CAD build for the part. Positions are in the model's coordinates, mm. Coordinates: 2 decimals unless noted, no trailing zeros. Order: outer loops, then holes, each group sorted by start corner. A loop starts at its lowest first (then second) coordinate and runs counter-clockwise, first axis right, second up. Notation, with made-up numbers: M -21,89.25 L 19,89.25 A27 ccw 19,107.25 Z; hole C 2,-39 d11. An arc over 180 degrees is marked long. Write item = value, one per line.
from build123d import *

# Parameters (mm, degrees)
SKETCH1_R           = 1.55
BOSS_EXTRUDE1_DEPTH = 5
FILLET1_R           = 1
SKETCH2_R           = 2.9
CUT_EXTRUDE1_DEPTH  = 3


with BuildPart() as part:
    # Sketch1 → Boss-Extrude1 (new body)
    with BuildSketch(Plane(origin=(0, 0, 0), x_dir=(1, 0, 0), z_dir=(0, 1, 0))):
        with BuildLine():
            ThreePointArc((-29.5, 4), (-33.5, 0), (-29.5, -4))
            ThreePointArc((-29.5, -4), (-16.900654795, -5.373538993), (-4.893229568, -9.429626812))
            ThreePointArc((-4.893229568, -9.429626812), (14.756477238, -11.986867848), (32.328427125, -2.828427125))
            ThreePointArc((32.328427125, -2.828427125), (32.328427125, 2.828427125), (26.671572875, 2.828427125))
            ThreePointArc((26.671572875, 2.828427125), (13.359489628, -4.109785544), (-1.526651892, -2.172481729))
            ThreePointArc((-1.526651892, -2.172481729), (-15.176874162, 2.438540137), (-29.5, 4))
        make_face()
        with Locations(Location((-29.5, 0, 0), (0, 0, 270))):
            Circle(SKETCH1_R, mode=Mode.SUBTRACT)
        with Locations(Location((29.5, 0, 0), (0, 0, 270))):
            Circle(SKETCH1_R, mode=Mode.SUBTRACT)
    extrude(amount=BOSS_EXTRUDE1_DEPTH)

    # Fillet1
    fillet1_edges = [part.edges().sort_by_distance(p)[0] for p in [
        (-16.900654795, 5, 5.373538993),
        (14.756477238, 5, 11.986867848),
        (32.328427125, 5, -2.828427125),
        (13.359489628, 5, 4.109785544),
        (-15.176874162, 5, -2.438540137),
        (13.359489628, 0, 4.109785544),
        (32.328427125, 0, -2.828427125),
        (14.756477238, 0, 11.986867848),
        (-16.900654795, 0, 5.373538993),
        (-33.5, 0, 0),
        (-15.176874162, 0, -2.438540137),
        (-33.5, 5, 0),
    ]]
    fillet(fillet1_edges, radius=FILLET1_R)

    # Sketch2 → Cut-Extrude1 (cut)
    with BuildSketch(Plane.XZ):
        with Locations(Location((29.5, 0, 0), (0, 0, 270))):
            Circle(SKETCH2_R)
        with Locations(Location((-29.5, 0, 0), (0, 0, 270))):
            Circle(SKETCH2_R)
    extrude(amount=-CUT_EXTRUDE1_DEPTH, mode=Mode.SUBTRACT)


solid = part.part
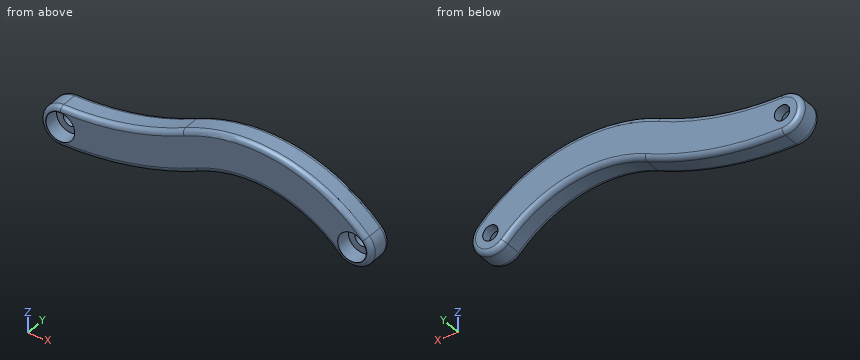
(1) Pin check, flat tips, straight feed: pin 1 Ø3 at (y, z) = (3.5, 10.5) entering from +X; pin 2 Ø3 at (y, z) = (4, 10) entering from +X; pin 3 Ø5 at (x, z) = (-29.5, 0) entering from -Y. Stop position of each tip, or through.
Evaluation:
pin_1 = 23.77
pin_2 = 24.73
pin_3 = 3
(2) Slice it at B-B, the plane z = 0. State how many separate pieces and enclosed holes the cut face has, then the cut area to 3 significant figures.
Evaluation:
separate_pieces = 4
enclosed_holes = 0
area = 134 mm²
(3) Slice it at A-A, the plane y = 1.65. Write the cut outline in (x, z).
Evaluation:
outline = M -29.5,-4 A66.47 ccw -1.53,2.17 A25 cw 26.67,-2.83 A4 ccw 32.33,2.83 A33 ccw -4.89,9.43 A58.47 cw -29.5,4 A4 ccw Z; hole C -29.5,0 d5.8; hole C 29.5,0 d5.8
(4) Wall check: line 1 (X direction, y = 3.4, z = 1); line 2 (Z direction, x = 27, y = 0.45); line 3 (Z direction, x = 30, y = 4.45). Give the ranges that are in metal, low to high. Write a range as from..to.
Evaluation:
line_1 = -33.37..-30.68, -28.32..-4.21, 21.74..28.32, 30.68..33.37
line_2 = -2.91..-1.47, 1.47..6.95
line_3 = -3.86..-1.47, 1.47..4.81
